Input: part model. Units: mm. Frame: model coordinates. A direction names the side the tool comes from. Coordinates: 2 decimals unless noted, no trailing zeros. Order: outer loops, then holes, each group sorted by start corner. A loop starts at its lowest first (then second) coordinate and runs counter-clockwise, first axis right, second up. Notation, with made-up numbers: (-13.5, 79.25) - (37.5, 79.25) arc R3 cw to (37.5, 84.25) - close; hole circle Ø5 at (3, -16). An arc over 180 degrees is marked (long way). Answer as CSV lines item,"result". Start each with the question number.
Item 1: Section D-D (z = 1.05). State how many separate pieces and enclosed holes the cut face has, and give its area (3 significant figures).
Item 2: Draft query along Y for faces 1 (the cylindrical face through (-76.275, -9.301, 2.028)), 2 (the flat face through (52.673, -12.293, 2.028)), 3 (the cylindrical face through (-25.68, -81.22, 2.03)). Return one class per face: +Y half, -Y half, draft (parallel to the pull), parting line (faces both ways), or undercut.
Item 3: Section C-C (x = 57). Output: boundary loops of the cut face in (y, z).
Item 4: First-contact query: pin 1 (2 mm diameter, centred on x = 65, z = 1, fed in from -Y); pin 2 (3 mm diameter, centred on x = 75, y = 0, fed in from +Z); pin 3 (1 mm diameter, centred on x = -54, z = 0.5, fed in from +Y); pin 4 (2 mm diameter, centred on y = -112.5, z = 1, fed in from +X). Flat tips, straight axial feed; report the tip coordinate or a pass-through.
Item 5: Access query for faces 4 (the cylindrical face through (70.213, -80.138, 2.028)), 5 (the flat face through (-53.072, -11.783, 2.028)). Directions: +Z, -Z, +X, -X, +Y, -Y. A direction counts if a zero-diameter tool reaches every point of the face in a straight line with its end or side. Return the directions, or none.
Item 6: Material intervals for line 1 along Y through (x, z) = (0, 2.4); line 2 along Y through (x, z) = (-75, 3.1); line 3 along Y through (x, z) = (52, 1.5), sorted ascending.
Item 7: Section B-B (y = -26). Output: boundary loops of the cut face in (x, z).
Item 8: Section A-A (x = 0). Output: boundary loops of the cut face in (y, z).
from build123d import *

# Parameters (mm, degrees)
SKETCH_1_R          = 2.55
EXTRUDE_1_DEPTH     = 4
EXTRUDE_2_DEPTH     = 4
FILLET_2_R          = 10
SKETCH_5_R          = 2.05
SKETCH_5_R_2        = 24.5
CUT_EXTRUDE_1_DEPTH = 5
CUT_EXTRUDE_2_DEPTH = 5
CUT_EXTRUDE_3_DEPTH = 25
FILLET_3_R          = 8
FILLET_4_R          = 5


with BuildPart() as part:
    # 草图1 → 凸台-拉伸1 (new body)
    with BuildSketch(Plane.XY):
        with BuildLine():
            Line((-85, -84), (85, -84))
            Line((85, -84), (85, 10))
            Line((85, 10), (48.019813619, 10))
            ThreePointArc((48.019813619, 10), (0, -49.05), (-48.019813619, 10))
            Line((-48.019813619, 10), (-85, 10))
            Line((-85, 10), (-85, -84))
        make_face()
        with Locations((75, 0)):
            Circle(SKETCH_1_R, mode=Mode.SUBTRACT)
        with Locations((-75, 0)):
            Circle(SKETCH_1_R, mode=Mode.SUBTRACT)
        with Locations((-75, -74)):
            Circle(SKETCH_1_R, mode=Mode.SUBTRACT)
        with Locations((75, -74)):
            Circle(SKETCH_1_R, mode=Mode.SUBTRACT)
    extrude(amount=EXTRUDE_1_DEPTH)

    # 草图2 → 凸台-拉伸2 (add)
    with BuildSketch(Plane.XY.offset(4)):
        with BuildLine():
            Line((-85, -84), (-19.866917685, -131.97323825))
            ThreePointArc((-19.866917685, -131.97323825), (0, -138.5), (19.866917685, -131.97323825))
            Line((19.866917685, -131.97323825), (85, -84))
            Line((85, -84), (-85, -84))
        make_face()
    extrude(amount=-EXTRUDE_2_DEPTH)

    # 圆角2
    fillet_2_edges = [part.edges().sort_by_distance(p)[0] for p in [
        (85, 10, 2),
        (-85, 10, 2),
    ]]
    fillet(fillet_2_edges, radius=FILLET_2_R)

    # 草图5 → 切除-拉伸1 (cut)
    with BuildSketch(Plane.XY.offset(4)):
        with Locations((15.367658663, -129.593394789)):
            Circle(SKETCH_5_R)
        with Locations((-28.982333984, -106.012085404)):
            Circle(SKETCH_5_R)
        with Locations((13.614675321, -79.394519807)):
            Circle(SKETCH_5_R)
        with Locations((0, -105)):
            Circle(SKETCH_5_R_2)
    extrude(amount=-CUT_EXTRUDE_1_DEPTH, mode=Mode.SUBTRACT)

    # 草图6 → 切除-拉伸2 (cut)
    with BuildSketch(Plane.XY.offset(4)):
        with BuildLine():
            Line((-67.126666667, 6.165275519), (-38.6187, -30.24067642))
            Line((-38.6187, -30.24067642), (38.6187, -30.24067642))
            Line((38.6187, -30.24067642), (67.126666667, 6.165275519))
            ThreePointArc((67.126666667, 6.165275519), (70.621230492, 8.990349136), (75, 10))
            Line((75, 10), (-75, 10))
            ThreePointArc((-75, 10), (-70.621230492, 8.990349136), (-67.126666667, 6.165275519))
        make_face()
    extrude(amount=-CUT_EXTRUDE_2_DEPTH, mode=Mode.SUBTRACT)

    # 草图7 → 切除-拉伸3 (cut)
    with BuildSketch(Plane.XY.offset(4)):
        Polygon((-77, -5.144778907), (-68.857155974, -4.600712255), (-43.359613768, -37.162217147), (-77, -70.354064895), align=None)
        with BuildLine():
            ThreePointArc((-36.942273764, -43.473795661), (-22.471434931, -52.437935811), (-6, -56.733609968))
            Line((-6, -56.733609968), (-6, -70.518120701))
            ThreePointArc((-6, -70.518120701), (-28.302069217, -84.408912655), (-34.654792832, -109.903604165))
            Line((-34.654792832, -109.903604165), (-74.514618659, -80.545175958))
            Line((-74.514618659, -80.545175958), (-36.942273764, -43.473795661))
        make_face()
        with BuildLine():
            ThreePointArc((34.654792832, -109.903604165), (28.302069217, -84.408912655), (6, -70.518120701))
            Line((6, -70.518120701), (6, -56.733609968))
            ThreePointArc((6, -56.733609968), (22.471434931, -52.437935811), (36.942273764, -43.473795661))
            Line((36.942273764, -43.473795661), (74.514618659, -80.545175958))
            Line((74.514618659, -80.545175958), (34.654792832, -109.903604165))
        make_face()
        Polygon((77, -70.354064895), (43.359613768, -37.162217147), (68.857155974, -4.600712255), (77, -5.144778907), align=None)
    extrude(amount=-CUT_EXTRUDE_3_DEPTH, mode=Mode.SUBTRACT)

    # 圆角3
    # the kernel refuses this fillet: 8 mm, written as the material it adds along each edge
    with BuildSketch(Plane(origin=(-6, -56.733609968, 4), x_dir=(0, -1, 0), z_dir=(0, 0, -1))) as fillet_3_piece_1:
        with BuildLine():
            CenterArc((6.791995106, 8), FILLET_3_R, 192.428379519, 77.571620481)
            ThreePointArc((-1.020531268, 6.278247502), (-0.422700314, 3.153357523), (0, 0))
            Line((0, 0), (6.791995106, 0))
        make_face()
    extrude(amount=4)
    with BuildSketch(Plane(origin=(-6, -70.518120701, 4), x_dir=(-0.9684273836136271, -0.2492958135774943, 0), z_dir=(0, 0, -1))) as fillet_3_piece_2:
        with BuildLine():
            CenterArc((6.207961727, 7.97462195), FILLET_3_R, 194.435845985, 70.999197637)
            Line((-1.539457342, 5.980255442), (0, 0))
            ThreePointArc((0, 0), (2.785623852, 0.111028967), (5.571247704, 0))
        make_face()
    extrude(amount=4)
    with BuildSketch(Plane(origin=(-34.654792832, -109.903604165, 4), x_dir=(-0.8051712910421941, 0.5930423189633656, 0), z_dir=(0, 0, -1))) as fillet_3_piece_3:
        with BuildLine():
            CenterArc((14.713311973, 8), FILLET_3_R, 157.435643024, 112.564356976)
            ThreePointArc((7.325719141, 11.069767442), (4.192460552, 5.184405893), (0, 0))
            Line((0, 0), (14.713311973, 0))
        make_face()
    extrude(amount=4)
    with BuildSketch(Plane(origin=(-74.514618659, -80.545175958, 4), x_dir=(0.711836432832338, 0.7023452803945736, 0), z_dir=(0, 0, -1)), Plane(origin=(74.514618659, -80.545175958, 4), x_dir=(-0.8051712910421942, -0.5930423189633655, 0), z_dir=(0, 0, -1))) as fillet_3_piece_4:
        with BuildLine():
            CenterArc((FILLET_3_R * 1.17108402506, FILLET_3_R), FILLET_3_R, 170.988669267, 99.011330733)
            Line((FILLET_3_R * 0.183426640042, FILLET_3_R * 1.15662978584), (0, 0))
            Line((0, 0), (FILLET_3_R * 1.17108402506, 0))
        make_face()
    extrude(amount=4)
    with BuildSketch(Plane(origin=(-36.942273764, -43.473795661, 4), x_dir=(-0.711836432832338, -0.7023452803945739, 0), z_dir=(0, 0, -1))) as fillet_3_piece_5:
        with BuildLine():
            CenterArc((6.907291952, -8), FILLET_3_R, 90, 78.47203041)
            ThreePointArc((-0.931326161, -6.401229823), (-0.374864481, -3.213825359), (0, 0))
            Line((0, 0), (6.907291952, 0))
        make_face()
    extrude(amount=4)
    with BuildSketch(Plane(origin=(43.359613768, -37.162217147, 4), x_dir=(0.616527551876007, 0.7873333333333332, 0), z_dir=(0, 0, -1)), Plane(origin=(-43.359613768, -37.162217147, 4), x_dir=(-0.7118364328323388, -0.7023452803945729, 0), z_dir=(0, 0, -1))) as fillet_3_piece_6:
        with BuildLine():
            CenterArc((FILLET_3_R * 0.891711791031, FILLET_3_R), FILLET_3_R, 186.552471372, 83.447528628)
            Line((-FILLET_3_R * 0.101755976712, FILLET_3_R * 0.885886922506), (0, 0))
            Line((0, 0), (FILLET_3_R * 0.891711791031, 0))
        make_face()
    extrude(amount=4)
    with BuildSketch(Plane(origin=(68.857155974, -4.600712255, 4), x_dir=(0.9977753031397176, -0.06666666666666672, 0), z_dir=(0, 0, -1)), Plane(origin=(-68.857155974, -4.600712255, 4), x_dir=(0.6165275518760065, -0.7873333333333337, 0), z_dir=(0, 0, -1))) as fillet_3_piece_7:
        with BuildLine():
            CenterArc((FILLET_3_R * 0.529020931448, FILLET_3_R), FILLET_3_R, 214.240445239, 55.759554761)
            Line((-FILLET_3_R * 0.297662660682, FILLET_3_R * 0.437332923922), (0, 0))
            Line((0, 0), (FILLET_3_R * 0.529020931448, 0))
        make_face()
    extrude(amount=4)
    with BuildSketch(Plane(origin=(77, -5.144778907, 4), x_dir=(0, -1, 0), z_dir=(0, 0, -1))) as fillet_3_piece_8:
        with BuildLine():
            CenterArc((FILLET_3_R * 0.935414346693, FILLET_3_R), FILLET_3_R, 183.822553729, 86.177446271)
            Line((-FILLET_3_R * 0.0623609564462, FILLET_3_R * 0.933333333333), (0, 0))
            Line((0, 0), (FILLET_3_R * 0.935414346693, 0))
        make_face()
    extrude(amount=4)
    with BuildSketch(Plane(origin=(77, -70.354064895, 4), x_dir=(0, 1, 0), z_dir=(0, 0, -1))) as fillet_3_piece_9:
        with BuildLine():
            CenterArc((FILLET_3_R * 2.39148377615, -FILLET_3_R), FILLET_3_R, 90, 134.61547034)
            Line((FILLET_3_R * 1.67964734332, -FILLET_3_R * 1.70234528039), (0, 0))
            Line((0, 0), (FILLET_3_R * 2.39148377615, 0))
        make_face()
    extrude(amount=4)
    with BuildSketch(Plane(origin=(-77, -70.354064895, 4), x_dir=(0, 1, 0), z_dir=(0, 0, -1))) as fillet_3_piece_10:
        with BuildLine():
            CenterArc((FILLET_3_R * 2.39148377615, FILLET_3_R), FILLET_3_R, 135.38452966, 134.61547034)
            Line((FILLET_3_R * 1.67964734332, FILLET_3_R * 1.70234528039), (0, 0))
            Line((0, 0), (FILLET_3_R * 2.39148377615, 0))
        make_face()
    extrude(amount=4)
    with BuildSketch(Plane(origin=(-77, -5.144778907, 4), x_dir=(0, -1, 0), z_dir=(0, 0, -1))) as fillet_3_piece_11:
        with BuildLine():
            CenterArc((FILLET_3_R * 0.935414346693, -FILLET_3_R), FILLET_3_R, 90, 86.177446271)
            Line((-FILLET_3_R * 0.0623609564462, -FILLET_3_R * 0.933333333333), (0, 0))
            Line((0, 0), (FILLET_3_R * 0.935414346693, 0))
        make_face()
    extrude(amount=4)
    with BuildSketch(Plane(origin=(6, -56.733609968, 4), x_dir=(0.9870448668515611, 0.16044447893892722, 0), z_dir=(0, 0, -1))) as fillet_3_piece_12:
        with BuildLine():
            CenterArc((6.806620819, 7.987559736), FILLET_3_R, 189.232696301, 77.571620481)
            Line((-1.089738116, 6.704003905), (0, 0))
            ThreePointArc((0, 0), (3.180325289, 0.08871463), (6.360650577, 0))
        make_face()
    extrude(amount=4)
    with BuildSketch(Plane(origin=(36.942273764, -43.473795661, 4), x_dir=(0.7118364328323379, -0.7023452803945738, 0), z_dir=(0, 0, -1))) as fillet_3_piece_13:
        with BuildLine():
            CenterArc((6.907291952, 8), FILLET_3_R, 191.52796959, 78.47203041)
            ThreePointArc((-0.931326161, 6.401229823), (-0.374864481, 3.213825359), (0, 0))
            Line((0, 0), (6.907291952, 0))
        make_face()
    extrude(amount=4)
    with BuildSketch(Plane(origin=(6, -70.518120701, 4), x_dir=(0, 1, 0), z_dir=(0, 0, -1))) as fillet_3_piece_14:
        with BuildLine():
            CenterArc((6.175223401, 8), FILLET_3_R, 199.000802363, 70.999197637)
            ThreePointArc((-1.388888729, 5.395348837), (-0.586920873, 2.725353475), (0, 0))
            Line((0, 0), (6.175223401, 0))
        make_face()
    extrude(amount=4)
    with BuildSketch(Plane(origin=(34.654792832, -109.903604165, 4), x_dir=(0.8051712910421941, 0.5930423189633658, 0), z_dir=(0, 0, -1))) as fillet_3_piece_15:
        with BuildLine():
            CenterArc((14.713311973, -8), FILLET_3_R, 90, 112.564356976)
            ThreePointArc((7.325719141, -11.069767442), (4.192460552, -5.184405893), (0, 0))
            Line((0, 0), (14.713311973, 0))
        make_face()
    extrude(amount=4)
    # the kernel refuses this fillet: 8 mm, written as the material it takes off along each edge
    with BuildSketch(Plane(origin=(-85, -84, -10.108598892), x_dir=(0, 1, 0), z_dir=(0, 0, 1))) as fillet_3_2_piece_1:
        with BuildLine():
            CenterArc((FILLET_3_R * 0.505429944614, -FILLET_3_R), FILLET_3_R, 90, 53.626801073)
            Line((-FILLET_3_R * 0.299741346428, -FILLET_3_R * 0.406957681037), (0, 0))
            Line((0, 0), (FILLET_3_R * 0.505429944614, 0))
        make_face()
    extrude(amount=24.217197785, mode=Mode.SUBTRACT)
    with BuildSketch(Plane(origin=(85, -84, -10.108598892), x_dir=(0, 1, 0), z_dir=(0, 0, 1))) as fillet_3_2_piece_2:
        with BuildLine():
            CenterArc((FILLET_3_R * 0.505429944614, FILLET_3_R), FILLET_3_R, 216.373198927, 53.626801073)
            Line((-FILLET_3_R * 0.299741346428, FILLET_3_R * 0.406957681037), (0, 0))
            Line((0, 0), (FILLET_3_R * 0.505429944614, 0))
        make_face()
    extrude(amount=24.217197785, mode=Mode.SUBTRACT)

    # 圆角4
    fillet_4_edges = [part.edges().sort_by_distance(p)[0] for p in [
        (71.293293442, -4.963838649, 2),
        (-71.293293442, -4.963838649, 2),
    ]]
    fillet(fillet_4_edges, radius=FILLET_4_R)


solid = part.part
Determined:
1,separate pieces,"1"
1,enclosed holes,"12"
1,area,"7,420 mm^2"
2,face 1,"undercut"
2,face 2,"+Y half"
2,face 3,"undercut"
3,outline,"(-104.62, 0) - (-93.45, 0) - (-93.45, 4) - (-104.62, 4) - close; (-63.26, 0) - (-50.62, 0) - (-50.62, 4) - (-63.26, 4) - close; (-19.74, 0) - (-6.77, 0) - (-6.77, 4) - (-19.74, 4) - close"
4,pin 1,"stops at y = -99.47"
4,pin 2,"passes through"
4,pin 3,"stops at y = -9.96"
4,pin 4,"stops at x = 47.66"
5,face 4,"+Z, -Z"
5,face 5,"+Z, -Z, +Y"
6,line 1,"y = -138.5 to -129.5, -80.5 to -49.05"
6,line 2,"y = -91.37 to -76.55, -71.45 to -56.51, -7.34 to -2.55, 2.55 to 10"
6,line 3,"y = -108.31 to -97.13, -58.33 to -45.69, -26.13 to -13.15"
7,outline,"(-85, 0) - (-77, 0) - (-77, 4) - (-85, 4) - close; (-52.1, 0) - (-41.94, 0) - (-41.94, 4) - (-52.1, 4) - close; (41.94, 0) - (52.1, 0) - (52.1, 4) - (41.94, 4) - close; (77, 0) - (85, 0) - (85, 4) - (77, 4) - close"
8,outline,"(-138.5, 0) - (-129.5, 0) - (-129.5, 4) - (-138.5, 4) - close; (-80.5, 0) - (-49.05, 0) - (-49.05, 4) - (-80.5, 4) - close"
